Check sheet for the modelled part. Datum: model origin and axes. Units: mm. Face numbers are marked on the shaded views. A direction names the side the tool comes from. Round coordinates to 2 decimals unless told otherwise and drop trailing zeros. Order: outer loops, then holes, each group sorted by start corner. A loop starts at its lowest first (then second) coordinate and runs counter-clockwise, first axis right, second up.
from build123d import *

# Parameters (mm, degrees)
BOX001_W     = 104.5
BOX001_H     = 102.5
BOX001_DEPTH = 42
BOX_W        = 114.5
BOX_H        = 112.5
BOX_DEPTH    = 40
FILLET_R     = 31
FILLET001_R  = 31
FILLET002_R  = 31
FILLET003_R  = 31
FILLET004_R  = 34
FILLET005_R  = 34
FILLET006_R  = 34


with BuildPart() as cubo001:
    # Box001 → Box001 (new body)
    with BuildSketch(Plane(origin=(5, 5, 0), x_dir=(1, 0, 0), z_dir=(0, 0, 1))):
        with Locations((52.25, 51.25)):
            Rectangle(BOX001_W, BOX001_H)
    extrude(amount=BOX001_DEPTH)


with BuildPart() as fillet006:
    # Box → Box (new body)
    with BuildSketch(Plane.XY):
        with Locations((57.25, 56.25)):
            Rectangle(BOX_W, BOX_H)
    extrude(amount=BOX_DEPTH)

    # Cut: cut Cubo001
    add(cubo001.part, mode=Mode.SUBTRACT)

    # Fillet
    fillet_edges = [fillet006.edges().sort_by_distance(p)[0] for p in [
        (5, 107.5, 20),
    ]]
    fillet(fillet_edges, radius=FILLET_R)

    # Fillet001
    fillet001_edges = [fillet006.edges().sort_by_distance(p)[0] for p in [
        (109.5, 107.5, 20),
    ]]
    fillet(fillet001_edges, radius=FILLET001_R)

    # Fillet002
    fillet002_edges = [fillet006.edges().sort_by_distance(p)[0] for p in [
        (5, 5, 20),
    ]]
    fillet(fillet002_edges, radius=FILLET002_R)

    # Fillet003
    fillet003_edges = [fillet006.edges().sort_by_distance(p)[0] for p in [
        (109.5, 5, 20),
    ]]
    fillet(fillet003_edges, radius=FILLET003_R)

    # Fillet004
    fillet004_edges = [fillet006.edges().sort_by_distance(p)[0] for p in [
        (0, 112.5, 20),
    ]]
    fillet(fillet004_edges, radius=FILLET004_R)

    # Fillet005
    fillet005_edges = [fillet006.edges().sort_by_distance(p)[0] for p in [
        (114.5, 112.5, 20),
    ]]
    fillet(fillet005_edges, radius=FILLET005_R)

    # Fillet006
    fillet006_edges = [fillet006.edges().sort_by_distance(p)[0] for p in [
        (114.5, 0, 20),
    ]]
    fillet(fillet006_edges, radius=FILLET006_R)


solid = fillet006.part
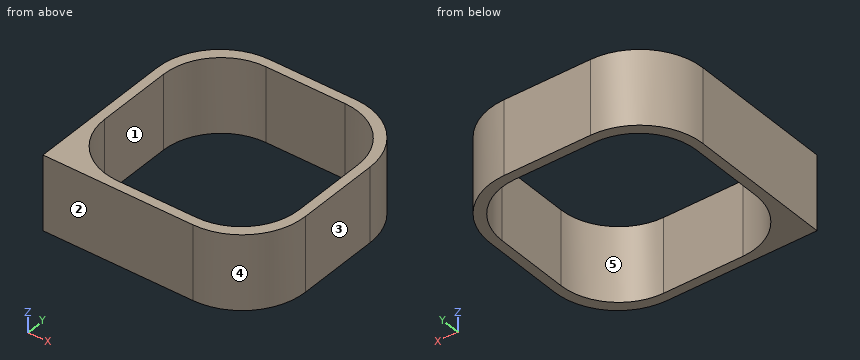
1) Set-up check for the marked faces 1 and 2: record each of +Z, -Z, +X, -X, +Y, -Y from which the full face is reachable in a straight line by a thin tool's end or side.
2) Gauge pin test, flat ends, axial feed: pin 1 (8 mm diameter, centred on y = 85, z = 10.5, fed in from -X); pin 2 (12 mm diameter, centred on y = 16, z = 8, fed in from +X); pin 3 (5 mm diameter, centred on x = 96.5, z = 9, fed in from +Y). Record the tip position at first contact, or that the pin passes through.
3) Sectioned sample at B-B on x = 70.5. Record the cut outline in (y, z).
4) Draft check along Y on the marked faces 3, 4 and 5. Enter one of: pulls with the +Y half, pulls with the -Y half, needs draft (parallel to the pull), parting line crosses it, or undercut.
5) Sectioned sample at A-A on y = 72. Record the cut outline in (x, z).
6) Sectioned sample at C-C on z = 13.5. Record the cut outline in (x, y).
7) Scan lines: line 1 (Y direction, x = 66, z = 4); line 2 (X direction, y = 61, z = 11); line 3 (Y direction, x = 86.5, z = 31). Record each from-to range of solid material in increasing order.
Values found:
1. face 1: +Z, -Z
1. face 2: +Z, -Z, +X, -X, -Y
2. pin 1: stops at x = 0.09
2. pin 2: stops at x = 112.31
2. pin 3: stops at y = 109.7
3. outline: (0, 0) - (5, 0) - (5, 40) - (0, 40) - close; (107.5, 0) - (112.5, 0) - (112.5, 40) - (107.5, 40) - close
4. face 3: needs draft
4. face 4: pulls with the -Y half
4. face 5: undercut
5. outline: (0, 0) - (5, 0) - (5, 40) - (0, 40) - close; (109.5, 0) - (114.5, 0) - (114.5, 40) - (109.5, 40) - close
6. outline: (0, 0) - (80.5, 0) arc R34 ccw to (114.5, 34) - (114.5, 78.5) arc R34 ccw to (80.5, 112.5) - (34, 112.5) arc R34 ccw to (0, 78.5) - close; hole (5, 36) arc R31 ccw to (36, 5) - (78.5, 5) arc R31 ccw to (109.5, 36) - (109.5, 76.5) arc R31 ccw to (78.5, 107.5) - (36, 107.5) arc R31 ccw to (5, 76.5) - close
7. line 1: y = 0 to 5, 107.5 to 112.5
7. line 2: x = 0 to 5, 109.5 to 114.5
7. line 3: y = 0.53 to 6.05, 106.45 to 111.97
